The listing builds one solid part. Answer for the finished solid, in the listing's coordinates (mm). A direction names the side the tool comes from. Give positions to 0.01 mm unless a question says otherwise; leave off trailing zeros. Loops run counter-clockwise (first coordinate to the right, second up) from the corner with the lowest first, then second, coordinate; pieces in that order, holes last. Notation, with made-up numbers: M -24,-12.75 L 23,-12.75 A15 cw 23,-0.75 Z; hole C -25,57.5 d5. An arc over 180 degrees is marked long. One line per item, written item: value. Start each with the question number.
Q1. A cutting plane is placed at D-D, the plane y = 15. Determine the outline of the cut face in (x, z).
Q2. The mould has two halves that part along Z. Classify faces 1 (the flat face through (0.253, 6.408, 11.842)), 2 (the flat face through (-2, 8.75, 12)), 3 (the flat face through (-0.51, 7.24, 10.18)): +Z half, -Z half, draft (parallel to the pull), parting line (faces both ways), or undercut.
Q3. For faces 4 (the flat face through (-3.67, 6.41, 11.02)), 5 (the flat face through (-1, 9.9, 3)), 6 (the flat face through (-2.984, 5.88, 19.776)), 7 (the flat face through (0, 7, 0)), determine the directions among +Z, -Z, +X, -X, +Y, -Y from which every point of the face is accessible in a straight line to the end or side of a thin tool.
Q4. A cutting plane is placed at B-B, the plane y = 6.75. Determine the outline of the cut face in (x, z).
Q5. Consider L1, parallel to Y at x = -1.5, z = 6.5; L2, parallel to X at y = 7.5, z = 12.75; L3, parallel to Y at x = -2.5, z = -2. Determine where each line is inside the solid, lowest interval first.
Q6. A cutting plane is placed at C-C, the plane z = 8.5. Determine the outline of the cut face in (x, y).
Q7. Flat-ended cylindrical pins translate along their axes: pin 1 (5 mm diameter, centred on x = -2.5, z = 7.5, fed in from -Y); pin 2 (1.9 mm diameter, centred on x = -2, z = 12.5, fed in from +Y); pin 3 (8 mm diameter, centred on y = 11, z = 10.5, fed in from -X). Find the tip coordinate at first contact, or state that the pin passes through.
Q8. A cutting plane is placed at A-A, the plane x = -1.25. Determine the outline of the cut face in (y, z), and give its area (3 significant figures).
from build123d import *

# Parameters (mm, degrees)
SKETCH1_R           = 3
BOSS_EXTRUDE1_DEPTH = 16.5
SKETCH2_R           = 3.7
BOSS_EXTRUDE2_DEPTH = 9.9
BOSS_EXTRUDE3_START = -8.75
BOSS_EXTRUDE3_DEPTH = 4.75
SKETCH4_R           = 0.2
BOSS_EXTRUDE4_DEPTH = 4
SKETCH5_W           = 2
SKETCH5_H           = 2
CUT_EXTRUDE1_DEPTH  = 20


with BuildPart() as part:
    # Sketch1 → Boss-Extrude1 (new body)
    with BuildSketch(Plane(origin=(0, 0, 0), x_dir=(1, 0, 0), z_dir=(0, 1, 0))):
        Circle(SKETCH1_R)
    extrude(amount=BOSS_EXTRUDE1_DEPTH)

    # Sketch2 → Boss-Extrude2 (add)
    with BuildSketch(Plane.XZ):
        Circle(SKETCH2_R)
    extrude(amount=-BOSS_EXTRUDE2_DEPTH)

    # Sketch3 → Boss-Extrude3 (add)
    with BuildSketch(Plane.XZ.offset(BOSS_EXTRUDE3_START)):
        with BuildLine():
            Line((-2.438116725, 2.783089441), (-4.934027826, 19.484747096))
            Line((-4.934027826, 19.484747096), (-0.977958543, 20.075945733))
            Line((-0.977958543, 20.075945733), (1.517952558, 3.374288078))
            ThreePointArc((1.517952558, 3.374288078), (-0.546858739, 3.659364087), (-2.438116725, 2.783089441))
        make_face()
    extrude(amount=BOSS_EXTRUDE3_DEPTH)

    # Sketch4 → Boss-Extrude4 (add)
    with BuildSketch(Plane(origin=(0, 16.5, 0), x_dir=(1, 0, 0), z_dir=(0, 1, 0))):
        Circle(SKETCH4_R)
    extrude(amount=BOSS_EXTRUDE4_DEPTH)

    # Sketch5 → Cut-Extrude1 (cut)
    with BuildSketch(Plane(origin=(-2.955993184, 0, 19.780346415), x_dir=(0.989017321, 0, 0.147799659), z_dir=(-0.147799659, 0, 0.989017321))):
        with Locations((0, 7.25)):
            Rectangle(SKETCH5_W, SKETCH5_H)
    extrude(amount=-CUT_EXTRUDE1_DEPTH, mode=Mode.SUBTRACT)


solid = part.part
Answer block:
1. outline: C 0,0 d6
2. face 1: +Z half
2. face 2: draft
2. face 3: undercut
3. face 4: -X, +Y, -Y
3. face 5: +Y
3. face 6: +Z, -X, +Y, -Y
3. face 7: none
4. outline: M -4.93,19.48 L -2.44,2.78 A3.7 ccw long 1.52,3.37 L -0.98,20.08 L -1.97,19.93 L 0.99,0.15 L -0.99,-0.15 L -3.95,19.63 Z
5. L1: 4 to 6.25, 8.25 to 8.75
5. L2: -3.93 to -2.92, -0.89 to 0.12
5. L3: 0 to 9.9
6. outline: M -3.29,4 L 0.75,4 L 0.75,8.75 L -3.29,8.75 Z; hole M -2.28,6.25 L -0.26,6.25 L -0.26,8.25 L -2.28,8.25 Z
7. pin 1: y = 4
7. pin 2: y = 8.75
7. pin 3: x = -4.09
8. outline: M 0,-3.48 L 9.9,-3.48 L 9.9,-2.73 L 16.5,-2.73 L 16.5,2.73 L 9.9,2.73 L 9.9,3.48 L 8.75,3.48 L 8.75,20.04 L 4,20.04 L 4,3.48 L 0,3.48 Z; hole M 6.25,1.6 L 8.25,1.6 L 8.25,15.13 L 6.25,15.13 Z
8. area: 157 mm^2
